Autodesk Inventor part; units mm, degrees
ref_plane "YZ Plane" through (0, 0, 0) normal (1, 0, 0) x (0, 1, 0)
ref_plane "XZ Plane" through (0, 0, 0) normal (0, 1, 0) x (-1, 0, 0)
ref_plane "XY Plane" through (0, 0, 0) normal (0, 0, 1) x (1, 0, 0)
sketch "Sketch1" plane through (0, 0, 0) normal (0, 0, 1) x (1, 0, 0)
  line L0 (-30, -30) -> (30, -30)
  line L1 (30, -30) -> (30, 30)
  line L2 (30, 30) -> (-30, 30)
  line L3 (-30, 30) -> (-30, -30)
  line L4 (-30, -30) -> (30, 30) construction
  line L5 (30, -30) -> (-30, 30) construction
  line L6 (15.1, -15.1) -> (-15.1, -15.1)
  line L7 (-15.1, -15.1) -> (-15.1, 15.1)
  line L8 (-15.1, 15.1) -> (15.1, 15.1)
  line L9 (15.1, 15.1) -> (15.1, -15.1)
  line L10 (15.1, -15.1) -> (-15.1, 15.1) construction
  line L11 (-15.1, -15.1) -> (15.1, 15.1) construction
  circle A0 centre (-23, -23) radius 2.75
  circle A1 centre (23, -23) radius 2.75
  circle A2 centre (23, 23) radius 2.75
  circle A3 centre (-23, 23) radius 2.75
  line L12 (25.75, 25.75) -> (-25.75, 25.75) construction
  line L13 (-25.75, 25.75) -> (-25.75, -25.75) construction
  line L14 (-25.75, -25.75) -> (25.75, -25.75) construction
  line L15 (25.75, -25.75) -> (25.75, 25.75) construction
  line L16 (25.75, 25.75) -> (-25.75, -25.75) construction
  line L17 (-25.75, 25.75) -> (25.75, -25.75) construction
  line L18 (23, 23) -> (-23, 23) construction
  line L19 (-23, 23) -> (-23, -23) construction
  line L20 (-23, -23) -> (23, -23) construction
  line L21 (23, -23) -> (23, 23) construction
  line L22 (23, 23) -> (-23, -23) construction
  line L23 (-23, 23) -> (23, -23) construction
  point P0 (0, 0)
  dimension "d172" = 30.2
  dimension "d190" = 5.5
  dimension "d191" = 46
  dimension "d192" = 60
extrude "Plate5" add sketch "Sketch1" along normal blind 3
fillet "Corner Round1" radius 2 4 edges at (30, 30, 1.5) (-30, 30, 1.5) (-30, -30, 1.5) (30, -30, 1.5)
fillet "Corner Round2" radius 1 4 edges at (-15.1, 15.1, 1.5) (-15.1, -15.1, 1.5) (15.1, -15.1, 1.5) (15.1, 15.1, 1.5)
properties part number "SLM 1425 FDS Way FLANGE" material "Stainless Steel"
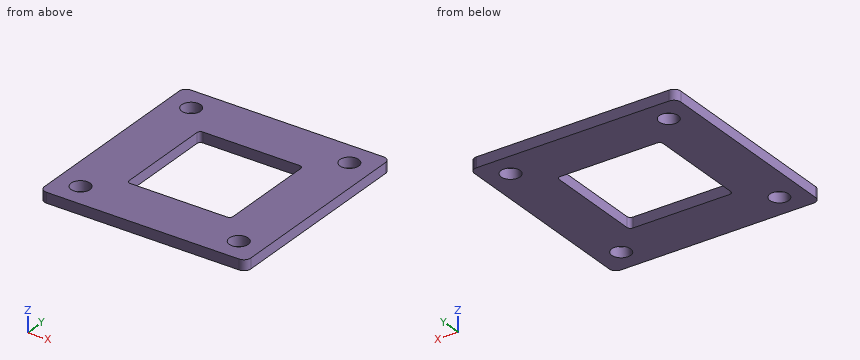
Verification items for the finished model (mm, model axes). Give positions to 0.01 mm unless a question says otherwise; leave off trailing zeros. Loops run counter-clockwise (first coordinate to the right, second up) from the corner with the lowest first, then second, coordinate; pieces in that order, holes last.
1. Cross-section at C-C on z = 0.5. Record the cut outline in (x, y), and give its area (3 significant figures).
Derived:
outline: (-30, -28) arc R2 ccw to (-28, -30) - (28, -30) arc R2 ccw to (30, -28) - (30, 28) arc R2 ccw to (28, 30) - (-28, 30) arc R2 ccw to (-30, 28) - close; hole circle Ø5.5 at (-23, -23); hole circle Ø5.5 at (-23, 23); hole (-15.1, -14.1) arc R1 ccw to (-14.1, -15.1) - (14.1, -15.1) arc R1 ccw to (15.1, -14.1) - (15.1, 14.1) arc R1 ccw to (14.1, 15.1) - (-14.1, 15.1) arc R1 ccw to (-15.1, 14.1) - close; hole circle Ø5.5 at (23, -23); hole circle Ø5.5 at (23, 23)
area: 2,590 mm2
2. Material ranges on probe 1 along Y at (x, z) = (23, 1.9); probe 2 along X at (y, z) = (-8, 1.7); probe 3 along Y at (x, z) = (-24, 0.45), recorded low to high.
Derived:
probe 1: y = -30 to -25.75, -20.25 to 20.25, 25.75 to 30
probe 2: x = -30 to -15.1, 15.1 to 30
probe 3: y = -30 to -25.56, -20.44 to 20.44, 25.56 to 30
3. Cross-section at A-A on y = 23. Record the cut outline in (x, z), and give its area (3 significant figures).
Derived:
outline: (-30, 0) - (-25.75, 0) - (-25.75, 3) - (-30, 3) - close; (-20.25, 0) - (20.25, 0) - (20.25, 3) - (-20.25, 3) - close; (25.75, 0) - (30, 0) - (30, 3) - (25.75, 3) - close
area: 147 mm2
4. Cross-section at B-B on x = 8.5. Record the cut outline in (y, z).
Derived:
outline: (-30, 0) - (-15.1, 0) - (-15.1, 3) - (-30, 3) - close; (15.1, 0) - (30, 0) - (30, 3) - (15.1, 3) - close
